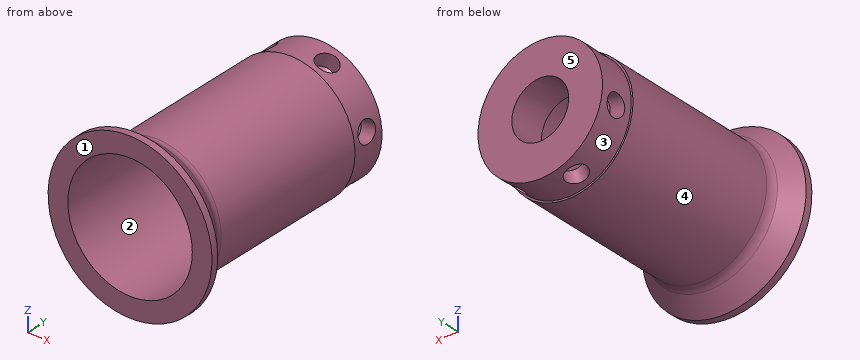
```python
from build123d import *

# Parameters (mm, degrees)
SKETCH2_R         = 13.890625
EXTRUDE2_DEPTH    = 44.196
CIRPATTERN1_COUNT = 6
SKETCH5_R         = 6.35
EXTRUDE3_DEPTH    = 53.3875


with BuildPart() as part:
    # Sketch1 → Revolve1 (revolve)
    with BuildSketch(Plane(origin=(0, 0, 0), x_dir=(0, 0, -1), z_dir=(1, 0, 0))):
        with BuildLine():
            Line((-18.288, 0), (-18.288, 1.5875))
            Line((-18.288, 1.5875), (-15.031387054, 5.464420173))
            ThreePointArc((-15.031387054, 5.464420173), (-14.479262782, 6.419853295), (-14.2875, 7.506555048))
            Line((-14.2875, 7.506555048), (-14.2875, 44.45))
            Line((-14.2875, 44.45), (-13.890625, 44.45))
            Line((-13.890625, 44.45), (-13.890625, 52.3875))
            Line((-13.890625, 52.3875), (0, 52.3875))
            Line((0, 52.3875), (0, 0))
            Line((0, 0), (-18.288, 0))
        make_face()
    revolve(axis=Axis((0, 52.3875, 0), (0, -1, 0)))

    # Sketch2 → Extrude2 (cut)
    with BuildSketch(Plane.XZ):
        Circle(SKETCH2_R)
    extrude(amount=-EXTRUDE2_DEPTH, mode=Mode.SUBTRACT)

    # Sketch4 → 3/16 (0.1875) Diameter Hole1 (revolve, cut)
    with BuildSketch(Plane(origin=(13.702535491, 48.41875, 2.278153639), x_dir=(0.164006561, 0, -0.986459248), z_dir=(0, 1, 0))):
        Polygon((0, 0), (0, 4.732799349), (2.38125, 3.302), (2.38125, 0), align=None)
    f_3_16_0_1875_diameter_hole1 = revolve(axis=Axis((19.966551716, 48.41875, 3.319595303), (-0.986459248, 0, -0.164006561)), mode=Mode.SUBTRACT)

    # CirPattern1: 3/16 (0.1875) Diameter Hole1 ×6 about axis
    cirpattern1_axis = Axis((0, 52.3875, 0), (0, 1, 0))
    for i in range(1, CIRPATTERN1_COUNT):
        add(f_3_16_0_1875_diameter_hole1.rotate(cirpattern1_axis, i * 360 / CIRPATTERN1_COUNT), mode=Mode.SUBTRACT)

    # Sketch5 → Extrude3 (cut, through all)
    with BuildSketch(Plane(origin=(0, 52.3875, 0), x_dir=(-1, 0, 0), z_dir=(0, 1, 0))):
        Circle(SKETCH5_R)
    extrude(amount=-EXTRUDE3_DEPTH, mode=Mode.SUBTRACT)


solid = part.part
```
For this review, take the finished solid that the model builds, in its own axes (mm). Face numbers are marked on the shaded views. A direction names the side the tool comes from. Round coordinates to 2 decimals unless told otherwise and drop trailing zeros. Write each loop counter-clockwise with the first axis right and the second up, starting at its lowest first coordinate (ties: lowest second). Pieces come first, ordered by that corner, then holes. Notation, with made-up numbers: (-27.5, 25) -> (-12.5, 25) arc R32 cw to (-12.5, 57) -> close; hole circle Ø11 at (22.5, 61). An arc over 180 degrees is marked (long way). Use one line per item in the form item = value.
1) Clearance check with flat-ended pins moving along their axes: pin 1 (1.5 mm diameter, centred on x = 8.5, y = 21.5, fed in from +Z); pin 2 (1.5 mm diameter, centred on y = 40.5, z = -8.5, fed in from -X); pin 3 (12 mm diameter, centred on x = -4.5, y = 39, fed in from +Z). State where each tip first meets the part, or that it passes through.
Found:
pin_1 = 12
pin_2 = -12
pin_3 = 14.29
2) Mouldability with a two-part tool opening along Z and no side actions: class the marked faces 1, 2 and 3 as +Z half, -Z half, draft (parallel to the pull), parting line (faces both ways), or undercut.
Found:
face_1 = draft
face_2 = undercut
face_3 = parting line
3) Take a section at B-B, the plane y = 9. Write out the cut boundary in (x, z) (1 decimal).
Found:
outline = circle Ø28.6 at (0, 0); hole circle Ø27.8 at (0, 0)
4) Tool access review of the marked faces 4 and 5: name each direction out of +Z, -Z, +X, -X, +Y, -Y from which nothing blocks a thin tool from reaching the whole face with its end or side.
Found:
face_4 = +Y
face_5 = +Z, -Z, +X, -X, +Y
5) To check wall thickness, follow L1, parallel to Z at x = 0, y = 49.75; L2, parallel to Z at x = 0, y = 22; L3, parallel to Y at x = 14, z = 1.5. State the ranges of each line that lie inside material, in increasing order. Write a range as from..to.
Found:
L1 = -13.89..-6.35, 6.35..13.89
L2 = -14.29..-13.89, 13.89..14.29
L3 = 0..44.45
